Read the model definition and answer for the solid it produces. Units are mm, in the model's axes. Coordinates: 2 decimals unless noted, no trailing zeros. Order: outer loops, then holes, each group sorted by start corner. A loop starts at its lowest first (then second) coordinate and runs counter-clockwise, first axis right, second up. Notation, with made-up numbers: (-24, 27.25) -> (15, 27.25) arc R11 ccw to (15, 48.25) -> close; hole circle Ø8 at (46, 7). An arc over 180 degrees is marked (long way). Answer in a Markdown table with one row per item.
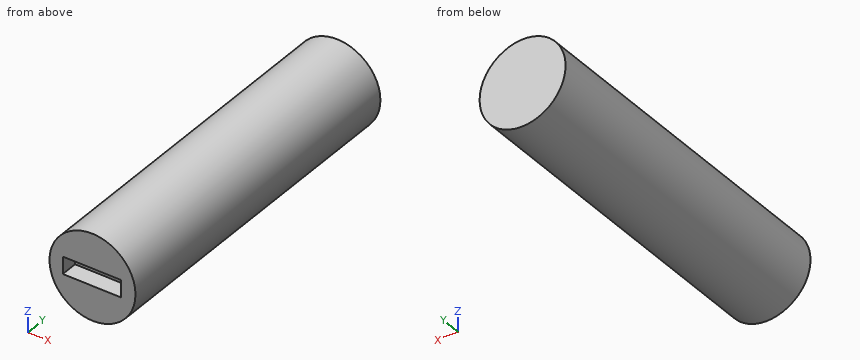
from build123d import *

# Parameters (mm, degrees)
F0_R     = 2.5
F1_DEPTH = 20
F2_W     = 3.388507
F2_H     = 1
F3_DEPTH = 1


with BuildPart() as f1:
    # F0 (on Front) → F1 (new body)
    with BuildSketch(Plane.XZ):
        Circle(F0_R)
    extrude(amount=F1_DEPTH)

    # F2 (on face) → F3 (cut)
    with BuildSketch(Plane.XZ.offset(20)):
        with Locations((-0.031836, 0)):
            Rectangle(F2_W, F2_H)
    extrude(amount=-F3_DEPTH, mode=Mode.SUBTRACT)


solid = f1.part
Q1. Given pin 1 (2 mm diameter, centred on y = -13.5, z = -1.5, fed in from +X); pin 2 (1.1 mm diameter, centred on x = -0.5, z = 0, fed in from -Y); pin 3 (1 mm diameter, centred on x = -1.5, y = -5.5, fed in from +Z); pin 4 (1 mm diameter, centred on y = -17, z = -1, fed in from -X), each flat-ended and moving along its own axis, determine where each tip first touches the part or whether it passes through.
Outcome:
| item | result |
|---|---|
| pin 1 | x = 2.45 |
| pin 2 | y = -20 |
| pin 3 | z = 2.29 |
| pin 4 | x = -2.45 |
Q2. Consider line 1 (X direction, y = -3.25, z = 0.1); line 2 (Y direction, x = 1.2, z = -0.45); line 3 (X direction, y = -13, z = 0.95). Determine where each line is inside the solid, lowest interval first.
Outcome:
| item | result |
|---|---|
| line 1 | -2.5 to 2.5 |
| line 2 | -19 to 0 |
| line 3 | -2.31 to 2.31 |
Q3. The part is cut by section D-D (z = 1.8). Write down the section's boundary in (x, y), then the cut area to 3 significant figures.
Outcome:
| item | result |
|---|---|
| outline | (-1.73, -20) -> (1.73, -20) -> (1.73, 0) -> (-1.73, 0) -> close |
| area | 69.4 mm² |
Q4. The part is cut by section B-B (y = -12.5). Write down the section's boundary in (x, z).
Outcome:
| item | result |
|---|---|
| outline | circle Ø5 at (0, 0) |
Q5. The part is cut by section C-C (x = 0.3). Write down the section's boundary in (y, z), then the cut area to 3 significant figures.
Outcome:
| item | result |
|---|---|
| outline | (-20, -2.48) -> (0, -2.48) -> (0, 2.48) -> (-20, 2.48) -> (-20, 0.5) -> (-19, 0.5) -> (-19, -0.5) -> (-20, -0.5) -> close |
| area | 98.3 mm² |
Q6. The part is cut by section A-A (z = 0). Write down the section's boundary in (x, y), then the cut area to 3 significant figures.
Outcome:
| item | result |
|---|---|
| outline | (-2.5, -20) -> (-1.73, -20) -> (-1.73, -19) -> (1.66, -19) -> (1.66, -20) -> (2.5, -20) -> (2.5, 0) -> (-2.5, 0) -> close |
| area | 96.6 mm² |
